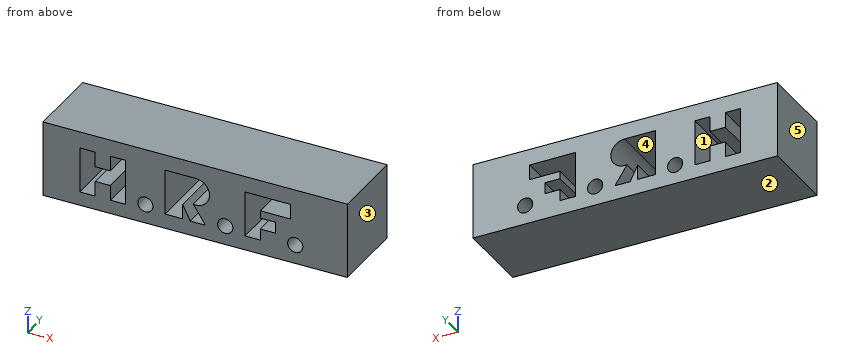
```python
from build123d import *

# Parameters (mm, degrees)
F0_W     = 508
F0_H     = 127
F0_R     = 12.7
F1_DEPTH = 127


with BuildPart() as f1:
    # F0 (on Front) → F1 (new body)
    with BuildSketch(Plane.XZ):
        with Locations((-362.030605, 31.507092)):
            Rectangle(F0_W, F0_H)
        Polygon((-554.435605, 67.223251), (-529.035605, 67.223251), (-529.035605, 41.823251), (-503.635605, 41.823251), (-503.635605, 67.223251), (-478.235605, 67.223251), (-478.235605, -8.976749), (-503.635605, -8.976749), (-503.635605, 16.423251), (-529.035605, 16.423251), (-529.035605, -8.976749), (-554.435605, -8.976749), align=None, mode=Mode.SUBTRACT)
        with Locations((-445.215605, 0)):
            Circle(F0_R, mode=Mode.SUBTRACT)
        with BuildLine():
            Line((-412.195605, -7.393757), (-412.195605, 68.716164))
            Line((-412.195605, 68.716164), (-361.10922, 68.716164))
            ThreePointArc((-361.10922, 68.716164), (-338.166668, 43.629273), (-365.198272, 23.01362))
            Line((-365.198272, 23.01362), (-344.88481, -7.859427))
            Line((-344.88481, -7.859427), (-370.28481, -7.859427))
            Line((-370.28481, -7.859427), (-382.873771, 17.540573))
            Line((-382.873771, 17.540573), (-382.873771, -7.393757))
            Line((-382.873771, -7.393757), (-412.195605, -7.393757))
        make_face(mode=Mode.SUBTRACT)
        with Locations((-311.86481, 0)):
            Circle(F0_R, mode=Mode.SUBTRACT)
        Polygon((-253.44481, -7.859427), (-278.84481, -7.859427), (-278.84481, 68.340573), (-202.645605, 67.992452), (-202.645605, 42.592452), (-253.445075, 42.824533), (-253.445075, 30.082439), (-228.04481, 30.082439), (-228.04481, 11.190573), (-253.44481, 11.190573), align=None, mode=Mode.SUBTRACT)
        with Locations((-195.02481, 0)):
            Circle(F0_R, mode=Mode.SUBTRACT)
    extrude(amount=F1_DEPTH)


solid = f1.part
```
Check sheet for the modelled part. Datum: model origin and axes. Units: mm. Face numbers are marked on the shaded views. A direction names the side the tool comes from. Coordinates: 2 decimals unless noted, no trailing zeros. Order: outer loops, then holes, each group sorted by start corner. A loop starts at its lowest first (then second) coordinate and runs counter-clockwise, first axis right, second up. Notation, with made-up numbers: (51, 63.5) -> (80, 63.5) arc R24 ccw to (80, 78.5) -> close; hole circle Ø4 at (-11.5, 61). An arc over 180 degrees is marked (long way). Write item = value, one per line. Start each with the question number.
1) Mould release check, pull along Z, two halves, no side actions. Record for the marked faces 1, 2 and 3: +Z half, -Z half, draft (parallel to the pull), parting line (faces both ways), or undercut.
2) Cross-section at B-B (z = 35). Enter the section's corners in (x, y).
3) Access from +Z, -Z, +X, -X, +Y, -Y to the whole of each face (thin tool, end or side, straight path). Record for the marked faces 4 and 5.
4) Cross-section at A-A (x = -548). Enter the section's corners in (y, z).
5) Go/stop test with a flat-tipped pin: P1, Ø10, axis at x = -526.5, z = 33, coming from the +Y side. Record where the tip stops, or that it passes through.
6) Cross-section at C-C (y = -24). State how many separate pieces and enclosed holes the cut face has, then the cut area to 3 significant figures.
7) Material ranges on L1, parallel to X at y = -80, z = 44; L2, parallel to X at y = -109, z = 56.5; L3, parallel to Z at x = -230, y = -98, recorded low to high.
Ans:
q1.face_1 = undercut
q1.face_2 = -Z half
q1.face_3 = draft
q2.outline = (-616.03, -127) -> (-554.44, -127) -> (-554.44, 0) -> (-616.03, 0) -> close; (-478.24, -127) -> (-412.2, -127) -> (-412.2, 0) -> (-478.24, 0) -> close; (-340.7, -127) -> (-278.84, -127) -> (-278.84, 0) -> (-340.7, 0) -> close; (-253.45, -127) -> (-108.03, -127) -> (-108.03, 0) -> (-253.45, 0) -> close
q3.face_4 = +Y, -Y
q3.face_5 = +Z, -Z, -X, +Y, -Y
q4.outline = (-127, -31.99) -> (0, -31.99) -> (0, -8.98) -> (-127, -8.98) -> close; (-127, 67.22) -> (0, 67.22) -> (0, 95.01) -> (-127, 95.01) -> close
q5.P1 = through
q6.separate_pieces = 1
q6.enclosed_holes = 6
q6.area = 50,000 mm²
q7.L1 = -616.03 to -554.44, -529.04 to -503.64, -478.24 to -412.2, -338.14 to -278.84, -202.65 to -108.03
q7.L2 = -616.03 to -554.44, -529.04 to -503.64, -478.24 to -412.2, -340.77 to -278.84, -202.65 to -108.03
q7.L3 = -31.99 to 11.19, 30.08 to 42.72, 68.12 to 95.01
